Geometry: final body of the model. Coordinates: model frame, mm. Face numbers are marked on the shaded views. A direction names the side the tool comes from. Give positions to 0.01 mm unless a question says otherwise; leave off trailing zeros. Loops run counter-clockwise (first coordinate to the right, second up) from the corner with the lowest first, then second, coordinate; pieces in that order, holes last.
from build123d import *

# Parameters (mm, degrees)
SKETCH1_W               = 24
SKETCH1_H               = 25
BOSS_EXTRUDE1_DEPTH     = 17
SKETCH2_W               = 20.2
SKETCH2_H               = 15
CUT_EXTRUDE1_DEPTH      = 33.526911935
BOSS_EXTRUDE2_DEPTH     = 17
SKETCH5_R               = 1.4
CUT_EXTRUDE5_DEPTH      = 37.304407446
BOSS_EXTRUDE3_DEPTH     = 2
CUT_EXTRUDE4_DEPTH      = 74.16252394
CUT_EXTRUDE4_DEPTH_BACK = 74.16252394
SKETCH7_R               = 2.05
BOSS_EXTRUDE4_DEPTH     = 16
CHAMFER1_SIZE           = 1
CHAMFER2_SIZE           = 8
CHAMFER2_SIZE2          = 13.856406461
FILLET1_R               = 10
SKETCH8_W               = 1.9
SKETCH8_H               = 25
BOSS_EXTRUDE5_DEPTH     = 5
CHAMFER5_SIZE           = 5
CHAMFER6_SIZE           = 10
FILLET5_R               = 3
SKETCH9_W               = 5
SKETCH9_H               = 20.312892552
CUT_EXTRUDE6_DEPTH      = 1
CHAMFER7_SIZE           = 1


# Some blends are built 0.0001 mm under size
with BuildPart() as part:
    # Sketch1 → Boss-Extrude1 (new body)
    with BuildSketch(Plane.XY):
        Rectangle(SKETCH1_W, SKETCH1_H)
    extrude(amount=BOSS_EXTRUDE1_DEPTH)

    # Sketch2 → Cut-Extrude1 (cut, through all)
    with BuildSketch(Plane(origin=(0, 12.5, 0), x_dir=(1, 0, 0), z_dir=(0, 1, 0))):
        with Locations((0, -7.5)):
            Rectangle(SKETCH2_W, SKETCH2_H)
    extrude(amount=-CUT_EXTRUDE1_DEPTH, mode=Mode.SUBTRACT)

    # Sketch3 → Boss-Extrude2 (add)
    with BuildSketch(Plane.XY.offset(17)):
        Polygon((-12, -12.5), (-20.1, -12.5), (-12, 2.5), align=None)
        Polygon((12, -12.5), (20.1, -12.5), (12, 2.5), align=None)
    extrude(amount=-BOSS_EXTRUDE2_DEPTH)

    # Sketch5 → Cut-Extrude5 (cut, through all)
    with BuildSketch(Plane.XZ.offset(12.5)):
        with Locations(Location((-14.9, 7.5, 0), (0, 0, 270))):
            Circle(SKETCH5_R)
        with Locations(Location((14.9, 7.5, 0), (0, 0, 270))):
            Circle(SKETCH5_R)
    extrude(amount=-CUT_EXTRUDE5_DEPTH, mode=Mode.SUBTRACT)

    # Sketch6 → Boss-Extrude3 (add)
    with BuildSketch(Plane.XY.offset(17)):
        with BuildLine():
            Line((12, 12.5), (40.935171065, 12.5))
            Line((40.935171065, 12.5), (40.935171065, 18.357473763))
            Line((40.935171065, 18.357473763), (36.855912663, 22.32654969))
            ThreePointArc((36.855912663, 22.32654969), (6.329925709, 17.315872383), (0, 47.595813056))
            Line((0, 47.595813056), (0, 58.207101621))
            Line((0, 58.207101621), (-8.6, 58.207101621))
            Line((-8.6, 58.207101621), (-8.6, 53.667646312))
            Line((-8.6, 53.667646312), (-12, 43.559109862))
            Line((-12, 43.559109862), (-12, 12.5))
            Line((-12, 12.5), (12, 12.5))
        make_face()
    extrude(amount=-BOSS_EXTRUDE3_DEPTH)

    # Sketch4 → Cut-Extrude4 (cut, two sides: drawn at the far end of the back side and taken through both)
    with BuildSketch(Plane(origin=(0, 0, 0), x_dir=(1, 0, 0), z_dir=(0, 1, 0)).offset(-CUT_EXTRUDE4_DEPTH_BACK)):
        Polygon((-8.6, -17), (-20.1, -17), (-20.1, -10.5), align=None)
    extrude(amount=CUT_EXTRUDE4_DEPTH + CUT_EXTRUDE4_DEPTH_BACK, mode=Mode.SUBTRACT)

    # Sketch7 → Boss-Extrude4 (add)
    with BuildSketch(Plane(origin=(0, 0, 15), x_dir=(-1, 0, 0), z_dir=(0, 0, -1))):
        with Locations(Location((-37.6, 16.9, 0), (0, 0, 180))):
            Circle(SKETCH7_R)
        with Locations(Location((5.4, 54.9, 0), (0, 0, 180))):
            Circle(SKETCH7_R)
    extrude(amount=BOSS_EXTRUDE4_DEPTH)

    # Chamfer1
    chamfer1_edges = [part.edges().sort_by_distance(p)[0] for p in [
        (-14.9, -12.5, 8.9),
        (14.9, -12.5, 8.9),
    ]]
    chamfer(chamfer1_edges, length=CHAMFER1_SIZE)

    # Chamfer2
    chamfer2_edges = [part.edges().sort_by_distance(p)[0] for p in [
        (12, 12.5, 16),
    ]]
    chamfer2_side = [part.faces().sort_by_distance(p)[0] for p in [
        (12, 7.5, 8.5),
    ]]
    chamfer(chamfer2_edges, length=CHAMFER2_SIZE, length2=CHAMFER2_SIZE2, reference=chamfer2_side[0])

    # Fillet1
    # the kernel refuses this fillet: 10 mm, written as the material it adds along each edge
    with BuildSketch(Plane(origin=(12, 4.5, 15), x_dir=(0.8660254037844397, 0.4999999999999979, 0), z_dir=(0, 0, 1))) as fillet1_piece_1:
        with BuildLine():
            CenterArc((4.625034769, -10), FILLET1_R, 90, 34.229107271)
            Line((-1, -1.732050808), (-1.112500695, -1.566691824))
            ThreePointArc((-1.112500695, -1.566691824), (-0.673205081, -0.766025404), (-0.173205081, 0.1))
            Line((-0.173205081, 0.1), (0, 0.2))
            Line((0, 0.2), (4.625034769, 0.2))
            Line((4.625034769, 0.2), (4.625034769, 0))
        make_face()
    extrude(amount=2)
    with BuildSketch(Plane(origin=(25.856406461, 12.5, 15), x_dir=(1, 0, 0), z_dir=(0, 0, 1))) as fillet1_piece_2:
        with BuildLine():
            CenterArc((FILLET1_R * 0.267949192431, -FILLET1_R), FILLET1_R, 90, 30)
            Line((-FILLET1_R * 0.232050807569, -FILLET1_R * 0.133974596216), (-FILLET1_R * 0.242050807569, -FILLET1_R * 0.11665408814))
            Line((-FILLET1_R * 0.242050807569, -FILLET1_R * 0.11665408814), (-FILLET1_R * 0.00535898384862, FILLET1_R * 0.02))
            Line((-FILLET1_R * 0.00535898384862, FILLET1_R * 0.02), (FILLET1_R * 0.267949192431, FILLET1_R * 0.02))
            Line((FILLET1_R * 0.267949192431, FILLET1_R * 0.02), (FILLET1_R * 0.267949192431, 0))
        make_face()
    extrude(amount=2)

    # Sketch8 → Boss-Extrude5 (add)
    with BuildSketch(Plane(origin=(0, 0, 15), x_dir=(-1, 0, 0), z_dir=(0, 0, -1))):
        with Locations((11.05, 25)):
            Rectangle(SKETCH8_W, SKETCH8_H)
    extrude(amount=BOSS_EXTRUDE5_DEPTH)

    # Chamfer5
    chamfer5_edges = [part.edges().sort_by_distance(p)[0] for p in [
        (-11.05, 37.5, 15),
    ]]
    chamfer(chamfer5_edges, length=CHAMFER5_SIZE - 0.0001)  # a hair under: the kernel refuses the full size

    # Chamfer6
    chamfer6_edges = [part.edges().sort_by_distance(p)[0] for p in [
        (-11.05, 12.5, 10),
    ]]
    chamfer(chamfer6_edges, length=CHAMFER6_SIZE - 0.0001)  # a hair under: the kernel refuses the full size

    # Fillet5
    fillet5_edges = [part.edges().sort_by_distance(p)[0] for p in [
        (40.935171065, 18.357473763, 16),
        (40.935171065, 12.5, 16),
        (-8.6, 58.207101621, 16),
        (0, 58.207101621, 16),
    ]]
    fillet(fillet5_edges, radius=FILLET5_R)

    # Sketch9 → Cut-Extrude6 (cut)
    with BuildSketch(Plane(origin=(-10.1, 0, 0), x_dir=(0, 0, -1), z_dir=(1, 0, 0))):
        with Locations((-7.5, 14.513989876)):
            Rectangle(SKETCH9_W, SKETCH9_H)
    extrude(amount=-CUT_EXTRUDE6_DEPTH, mode=Mode.SUBTRACT)

    # Chamfer7
    chamfer7_edges = [part.edges().sort_by_distance(p)[0] for p in [
        (-10.1, 10.9287218, 5),
        (-10.1, 4.3575436, 7.5),
        (-10.1, 20.9287718, 10),
    ]]
    chamfer(chamfer7_edges, length=CHAMFER7_SIZE - 0.0001)  # a hair under: the kernel refuses the full size


solid = part.part
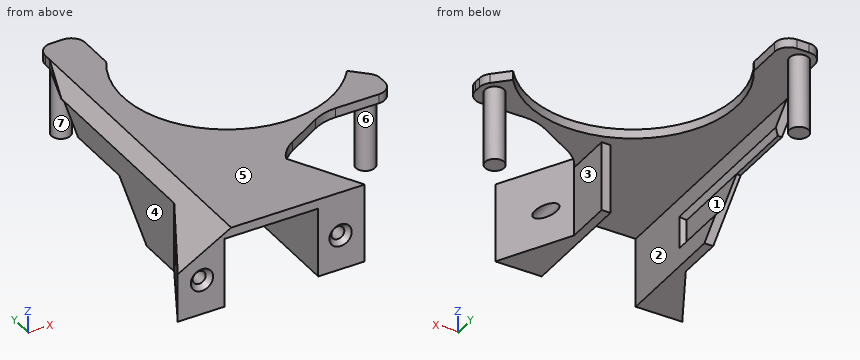
Item 1: Section query A-A on x = -14.9. Return loops of the section in (y, z), plus the area to 3 significant figures.
Values follow:
outline: (-12.5, 0) - (-2.87, 0) - (-2.87, 6.1) - (-11.5, 6.1) - (-12.5, 5.1) - close; (-12.5, 9.9) - (-11.5, 8.9) - (-2.87, 8.9) - (-2.87, 13.44) - (-12.5, 13.44) - close
area: 101 mm2
Item 2: Section query D-D on x = 14.9. Return loops of the section in (y, z), plus the area to 3 significant figures.
Values follow:
outline: (-12.5, 0) - (-2.87, 0) - (-2.87, 6.1) - (-11.5, 6.1) - (-12.5, 5.1) - close; (-12.5, 9.9) - (-11.5, 8.9) - (-2.87, 8.9) - (-2.87, 17) - (-12.5, 17) - close; (6.07, 15) - (13.77, 15) - (13.77, 17) - (6.07, 17) - close
area: 151 mm2
Item 3: Ray query, probe 1 along X at (y, z) = (8, 7.5); probe 2 along Z at (x, y) = (14.9, -6); probe 3 along X at (y, z) = (-6.5, 7.75). Return the intervals inside material, ascending.
Values follow:
probe 1: x = -12 to -11.1, 10.1 to 12
probe 2: z = 0 to 6.1, 8.9 to 17
probe 3: x = -16.86 to -16.28, -13.52 to -10.1, 10.1 to 13.52, 16.28 to 16.86
Item 4: Set-up query: the marked faces 1, 2, 3 and 4. Return all of +Z, -Z, +X, -X, +Y, -Y with unobstructed straight access to the full face (end or side cutting, diameter ignored); none if empty.
Values follow:
face 1: +Y
face 2: -Z, +Y, -Y
face 3: -Z, +X, +Y
face 4: +Z, -Z, -X, +Y
Item 5: Section query C-C on y = -5.5. Return loops of the section in (x, z).
Values follow:
outline: (-16.32, 0) - (-10.1, 0) - (-10.1, 15) - (10.1, 15) - (10.1, 0) - (16.32, 0) - (16.32, 17) - (-8.6, 17) - (-16.32, 12.64) - close; hole circle Ø2.8 at (-14.9, 7.5); hole circle Ø2.8 at (14.9, 7.5)
Item 6: Draft query along X for the marked faces 5, 6 and 7. Return one class per face: +X half, -X half, draft (parallel to the pull), parting line (faces both ways), or undercut.
Values follow:
face 5: draft
face 6: undercut
face 7: parting line
Item 7: Section query B-B on z = 13. Return loops of the section in (x, y).
Values follow:
outline: (-15.68, -12.5) - (-10.1, -12.5) - (-10.1, 40.5) - (-12, 40.5) - (-12, 2.5) - (-15.68, -4.31) - close; circle Ø4.1 at (-5.4, 54.9); (10.1, -12.5) - (20.1, -12.5) - (12, 2.5) - (12, 12.5) - (10.1, 12.5) - close; circle Ø4.1 at (37.6, 16.9)
Item 8: Pin query (flat end, axial travel): pin 1 (8 mm diameter, centred on y = 47, z = 2.5, fed in from -X); pin 2 (0.8 mm diameter, centred on y = 54.5, z = 16.5, fed in from -X); pin 3 (2.5 mm diameter, centred on y = 17, z = 8, fed in from +X); pin 4 (8 mm diameter, centred on x = 16.5, z = 10.5, fed in from +Y). Return the tip coordinate at first contact, or that it passes through.
Values follow:
pin 1: passes through
pin 2: stops at x = -8.6
pin 3: stops at x = 39.65
pin 4: stops at y = 1.57
